```python
from build123d import *

# Parameters (mm, degrees)
SKETCH1_R                       = 20
BOSS_EXTRUDE1_DEPTH             = 68
SKETCH2_R                       = 4
CUT_EXTRUDE1_DEPTH              = 10
CHAMFER1_SIZE                   = 3
CUT_EXTRUDE3_START              = -12
SKETCH5_R                       = 20
SKETCH5_R_2                     = 19
CUT_EXTRUDE3_DEPTH              = 2
LPATTERN1_COUNT                 = 15
LPATTERN1_PITCH                 = 3
CHAMFER2_SIZE                   = 1
BOSS_EXTRUDE2_REACH             = 83.388
BOSS_EXTRUDE2_END_RADIUS        = 20
SKETCH6_W                       = 8.4
SKETCH6_H                       = 10.5
BOSS_EXTRUDE2_DIRECTION_2_DEPTH = 5.5
CUT_EXTRUDE4_DEPTH              = 10.1


with BuildPart() as part:
    # Sketch1 → Boss-Extrude1 (new body)
    with BuildSketch(Plane.XY):
        Circle(SKETCH1_R)
    extrude(amount=BOSS_EXTRUDE1_DEPTH)

    # Sketch2 → Cut-Extrude1 (cut)
    with BuildSketch(Plane.XY.offset(68)):
        Circle(SKETCH2_R)
    extrude(amount=-CUT_EXTRUDE1_DEPTH, mode=Mode.SUBTRACT)

    # Chamfer1
    chamfer1_edges = [part.edges().sort_by_distance(p)[0] for p in [
        (-20, 0, 0),
        (-20, 0, 68),
    ]]
    chamfer(chamfer1_edges, length=CHAMFER1_SIZE)

    # Sketch5 → Cut-Extrude3 (cut)
    with BuildSketch(Plane.XY.offset(68).offset(CUT_EXTRUDE3_START)):
        Circle(SKETCH5_R)
        Circle(SKETCH5_R_2, mode=Mode.SUBTRACT)
    cut_extrude3 = extrude(amount=-CUT_EXTRUDE3_DEPTH, mode=Mode.SUBTRACT)

    # LPattern1: Cut-Extrude3 ×15
    with Locations(*[(0, 0, -i * LPATTERN1_PITCH) for i in range(1, LPATTERN1_COUNT)]):
        add(cut_extrude3, mode=Mode.SUBTRACT)

    # Chamfer2
    chamfer2_edges = [part.edges().sort_by_distance(p)[0] for p in [
        (-4, 0, 68),
    ]]
    chamfer(chamfer2_edges, length=CHAMFER2_SIZE)

    # Boss-Extrude2: up to this cylinder (the profile starts outside it)
    boss_extrude2_end = Plane(origin=(0, 0, 5.9), z_dir=(0, 0, -1)) * Cylinder(BOSS_EXTRUDE2_END_RADIUS, 207.776, mode=Mode.PRIVATE)
    # Sketch6 → Boss-Extrude2 (add, up to the surface)
    with BuildSketch(Plane.ZY.offset(20), mode=Mode.PRIVATE) as boss_extrude2_sk1:
        with Locations((5.9, 5.25)):
            Rectangle(SKETCH6_W, SKETCH6_H)
    boss_extrude2_tool1 = extrude(boss_extrude2_sk1.sketch, amount=-BOSS_EXTRUDE2_REACH, mode=Mode.PRIVATE) - boss_extrude2_end
    add(boss_extrude2_tool1.solids().sort_by_distance((-20, 5.25, 5.9))[0])
    # Sketch6 → Boss-Extrude2 (add, up to the surface)
    with BuildSketch(Plane.ZY.offset(20), mode=Mode.PRIVATE) as boss_extrude2_sk2:
        with Locations((5.9, -5.25)):
            Rectangle(SKETCH6_W, SKETCH6_H)
    boss_extrude2_tool2 = extrude(boss_extrude2_sk2.sketch, amount=-BOSS_EXTRUDE2_REACH, mode=Mode.PRIVATE) - boss_extrude2_end
    add(boss_extrude2_tool2.solids().sort_by_distance((-20, -5.25, 5.9))[0])

    # Sketch6 → Boss-Extrude2 direction 2 (add)
    with BuildSketch(Plane.ZY.offset(20)):
        with Locations((5.9, 5.25)):
            Rectangle(SKETCH6_W, SKETCH6_H)
        with Locations((5.9, -5.25)):
            Rectangle(SKETCH6_W, SKETCH6_H)
    extrude(amount=BOSS_EXTRUDE2_DIRECTION_2_DEPTH)

    # Sketch7 → Cut-Extrude4 (cut)
    with BuildSketch(Plane.XY):
        with BuildLine():
            Line((-22.963285915, 10.5), (-25.5, 10.5))
            Line((-25.5, 10.5), (-25.5, 0))
            Line((-25.5, 0), (-25.25, 0))
            ThreePointArc((-25.25, 0), (-24.671699063, 5.373059215), (-22.963285915, 10.5))
        make_face()
        with BuildLine():
            Line((-25.25, 0), (-25.5, 0))
            Line((-25.5, 0), (-25.5, -10.5))
            Line((-25.5, -10.5), (-22.963285915, -10.5))
            ThreePointArc((-22.963285915, -10.5), (-24.671699063, -5.373059215), (-25.25, 0))
        make_face()
    extrude(amount=CUT_EXTRUDE4_DEPTH, mode=Mode.SUBTRACT)


solid = part.part
```
CAD build for the part. Positions are in the model's coordinates, mm. Coordinates: 2 decimals unless noted, no trailing zeros. Write each loop counter-clockwise with the first axis right and the second up, starting at its lowest first coordinate (ties: lowest second). Pieces come first, ordered by that corner, then holes. Notation, with made-up numbers: (24.5, -39) -> (58.5, -39) arc R20 ccw to (58.5, -28) -> close; hole circle Ø10 at (17, 10). An arc over 180 degrees is marked (long way). Use CSV: the item, a comma, the result in double quotes. Start each with the question number.
Item 1: Drop flat-ended pins along their axis: P1, Ø5, axis at x = -20.5, z = 4.5, coming from the -Y side; P2, Ø2, axis at x = 14.5, z = 26.5, coming from the +Y side; P3, Ø1.5, axis at y = 4, z = 9, coming from the +X side. Give the stop position or say it passes through.
Item 2: Band-saw the part on B-B, the plane z = 22. Write the cut outline in (x, y).
Item 3: Wall check: probe 1 along Y at (x, z) = (0, 63.5); probe 2 along Y at (x, z) = (-8.5, 13); probe 3 along X at (y, z) = (-7, 19.5). Give the ranges that are in metal, low to high.
Item 4: Two-plate mould, pull along Z, no slides. Class faces 1 (the cylindrical face through (-4.336, -19.524, 60.437)), 2 (the flat face through (4, -4, 68)), 3 (the cylindrical face through (8.767, -16.856, 43.014)): +Z half, -Z half, draft (parallel to the pull), parting line (faces both ways), or undercut.
Item 5: Band-saw the part on A-A, the plane z = 60.5. Write the cut outline in (x, y).
Response values:
1,P1,"stops at y = -10.5"
1,P2,"stops at y = 14.76"
1,P3,"stops at x = 19.73"
2,outline,"circle Ø38 at (0, 0)"
3,probe 1,"y = -20 to -4, 4 to 20"
3,probe 2,"y = -16.99 to 16.99"
3,probe 3,"x = -17.66 to 17.66"
4,face 1,"draft"
4,face 2,"+Z half"
4,face 3,"undercut"
5,outline,"circle Ø40 at (0, 0); hole circle Ø8 at (0, 0)"
